The listing builds one solid part. Answer for the finished solid, in the listing's coordinates (mm). Face numbers are marked on the shaded views. A direction names the side the tool comes from. Round coordinates to 2 decimals unless told otherwise and drop trailing zeros. Write each loop counter-clockwise with the first axis right and the second up, starting at its lowest first coordinate (ties: lowest second). Pieces come first, ordered by that corner, then holes. Notation, with made-up numbers: M 73.25,84.25 L 126.25,84.25 A19 ccw 126.25,117.25 Z; hole C 16,48.5 d10. An arc over 180 degrees is marked long. Put each result on its own line as item: value. Start each with the question number.
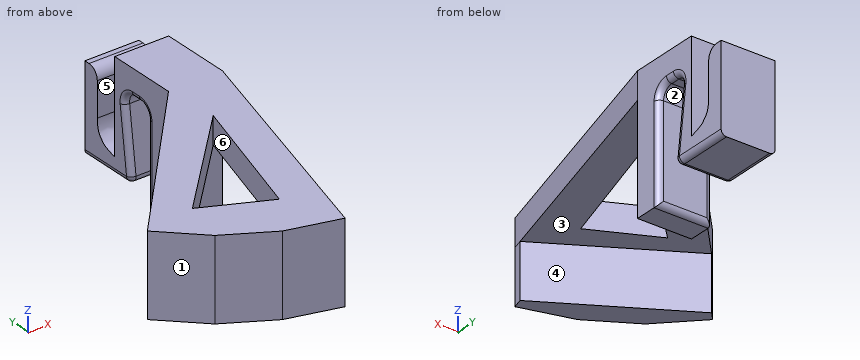
```python
from build123d import *

# Parameters (mm, degrees)
BOSS_EXTRUDE1_DEPTH = 10
BOSS_EXTRUDE2_DEPTH = 5
BOSS_EXTRUDE3_DEPTH = 10
FILLET1_R           = 2
FILLET2_R           = 1


with BuildPart() as part:
    # Sketch2 → Boss-Extrude1 (new body)
    with BuildSketch(Plane(origin=(0, 0, 0), x_dir=(0, 0, -1), z_dir=(1, 0, 0))):
        with BuildLine():
            Line((17, 13), (20, 13))
            Line((20, 13), (20, 20.212962963))
            Line((20, 20.212962963), (4, 20.212962963))
            Line((4, 20.212962963), (4, 19.212962963))
            ThreePointArc((4, 19.212962963), (4.585786438, 17.798749401), (6, 17.212962963))
            Line((6, 17.212962963), (12.34969837, 17.212962963))
            add(Edge.make_bspline(
                [(12.34969837, 17.212962963), (14.53461085, 17.212962963), (15.619631597, 15.872704948), (16.340899905, 15.502936293), (17, 13)],
                knots=[0, 0, 0, 0, 0.495488683, 1, 1, 1, 1], degree=3))
        make_face()
        Polygon((20, 11), (20, 13), (17, 13), (5, 13), (5, 11), align=None)
        with BuildLine():
            Line((20, 10.142183063), (20, 11))
            Line((20, 11), (5, 11))
            Line((5, 11), (18.86783628, 9.150955163))
            ThreePointArc((18.86783628, 9.150955163), (19.658724631, 9.389798946), (20, 10.142183063))
        make_face()
        Polygon((5, 11), (5, 13), (0, 13), (0, 0), (5, 0), (5, 3), (5, 5), align=None)
        Polygon((25, 5), (5, 5), (5, 3), (5, 0), (25, 0), align=None)
    extrude(amount=BOSS_EXTRUDE1_DEPTH)

    # Sketch4 → Boss-Extrude2 (add)
    with BuildSketch(Plane.XY):
        Polygon((10, 0), (-2.208590345, -45.563079458), (-11.867848608, -42.974889007), (-20.528102646, -37.974889007), (-27.599170458, -30.903821195), (0, 0), align=None)
        Polygon((-18.277381589, -29.621786509), (-6.470899787, -35.226395597), (0.864887029, -9.676755979), align=None, mode=Mode.SUBTRACT)
    extrude(amount=-BOSS_EXTRUDE2_DEPTH)

    # Sketch5 → Boss-Extrude3 (add)
    with BuildSketch(Plane(origin=(0, 0, -5), x_dir=(-1, 0, 0), z_dir=(0, 0, -1))):
        Polygon((2.208590345, -45.563079458), (11.867848608, -42.974889007), (20.528102646, -37.974889007), (27.599170458, -30.903821195), (26.266965075, -29.412101108), (1.690952255, -43.631227805), align=None)
    extrude(amount=BOSS_EXTRUDE3_DEPTH)

    # Fillet1
    fillet1_edges = [part.edges().sort_by_distance(p)[0] for p in [
        (5, 11, -5),
        (5, 5, -5),
    ]]
    fillet(fillet1_edges, radius=FILLET1_R)

    # Fillet2
    fillet2_edges = [part.edges().sort_by_distance(p)[0] for p in [
        (0, 15.177573013, -20),
        (0, 9.389798946, -19.658724631),
        (0, 9.924522419, -13.06608186),
        (10, 9.924522419, -13.06608186),
        (10, 9.389798946, -19.658724631),
        (5, 5, -25),
        (10, 15.177573013, -20),
        (0, 7.857816937, -5),
        (10, 7.857816937, -5),
        (0, 5, -16),
        (10, 5, -16),
        (0, 5.585786438, -5.585786438),
        (10, 5.585786438, -5.585786438),
        (0, 10.220402108, -5.682550737),
        (10, 10.220402108, -5.682550737),
    ]]
    fillet(fillet2_edges, radius=FILLET2_R)


solid = part.part
```
Item 1: Flat-ended cylindrical pins translate along their axes: pin 1 (4 mm diameter, centred on x = -23, z = -8, fed in from +Y); pin 2 (1.9 mm diameter, centred on x = 2.5, z = -8.5, fed in from -Y); pin 3 (5 mm diameter, centred on x = 1.5, y = -34.5, fed in from +Z); pin 4 (1.4 mm diameter, centred on x = 7, y = 8, fed in from -Z). Find the tip coordinate at first contact, or state that the pin passes through.
Item 2: Section A-A (y = -16) is taken. Give the vertices of the cut face in (x, z), and give its area (3 significant figures).
Item 3: Section B-B (x = -4) is taken. Give the vertices of the cut face in (y, z), and give its area (3 significant figures).
Item 4: Section D-D (z = -9.25) is taken. Count the separate pieces of the cut face and the enclosed holes in it, and give its area (3 significant figures).
Item 5: Section C-C (z = -22.25) is taken. Give the vertices of the cut face in (x, y), and give its area (3 significant figures).
Item 6: Consider line 1 along Y through (x, z) = (5.5, -21); line 2 along X through (y, z) = (-17, -1.25); line 3 along Z through (x, y) = (3.5, -1.5). Determine where each line is inside the solid, lowest interval first. Write a range as [from, to].
Item 7: Determine the mould class of the marked faces 1, 2 and 3 for opening direction Y: released by +Y, released by -Y, zero draft, split by the parting line, or undercut.
Item 8: Which of the six approach directions +Z, -Z, +X, -X, +Y, -Y give full straight-line access (tool end or side, diameter ignored) to the marked faces 4, 5 and 6?
Output values:
1. pin 1: stops at y = -30.15
1. pin 2: stops at y = 0
1. pin 3: stops at z = 0
1. pin 4: stops at z = -5
2. outline: M -14.29,-5 L -5.2,-5 L -5.2,0 L -14.29,0 Z; M -0.95,-5 L 5.71,-5 L 5.71,0 L -0.95,0 Z
2. area: 78.7 mm^2
3. outline: M -45.08,-15 L -42.3,-15 L -42.3,-5 L -26.62,-5 L -26.62,0 L -45.08,0 Z; M -14.75,-5 L -4.48,-5 L -4.48,0 L -14.75,0 Z
3. area: 172 mm^2
4. separate pieces: 4
4. enclosed holes: 0
4. area: 212 mm^2
5. outline: M 0,0 L 10,0 L 10,4 A1 ccw 9,5 L 1,5 A1 ccw 0,4 Z
5. area: 49.6 mm^2
6. line 1: y = [0, 5]
6. line 2: x = [-15.18, -6.16], [-1.24, 5.44]
6. line 3: z = [-5, 0]
7. face 1: released by -Y
7. face 2: undercut
7. face 3: zero draft
8. face 4: -Z, +X, +Y
8. face 5: +Z, +X, -X
8. face 6: +Z, -Z
